```python
from build123d import *

# Parameters (mm, degrees)
SKETCH1_W                    = 3.175
SKETCH1_H                    = 244
BASE_FLANGE1_DEPTH           = 15
EDGE_FLANGE1_STRIP_W         = 14.1732
EDGE_FLANGE1_STRIP_H         = 3.175
EDGE_FLANGE1_STRIP_CUT_DEPTH = 244
EDGE_FLANGE1_DEPTH           = 244


# Sheet-metal steps are written as plain solids
with BuildPart() as part:
    # Sketch1 → Base-Flange1 (new body)
    with BuildSketch(Plane(origin=(0, 0, 0), x_dir=(0, 0, -1), z_dir=(1, 0, 0))):
        with Locations((1.5875, 0)):
            Rectangle(SKETCH1_W, SKETCH1_H)
    extrude(amount=BASE_FLANGE1_DEPTH)

    # Edge-Flange1 strip (across the edge) → Edge-Flange1 strip cut (cut)
    with BuildSketch(Plane.XZ.offset(-122)):
        with Locations((-3.175, -1.5875)):
            Rectangle(EDGE_FLANGE1_STRIP_W, EDGE_FLANGE1_STRIP_H)
    extrude(amount=EDGE_FLANGE1_STRIP_CUT_DEPTH, mode=Mode.SUBTRACT)

    # Edge-Flange1 section (across the edge) → Edge-Flange1 (add)
    with BuildSketch(Plane.XZ.offset(-122)):
        with BuildLine():
            Line((0, 0.7366), (0, 11.825))
            Line((0, 11.825), (3.175, 11.825))
            Line((3.175, 11.825), (3.175, 0.7366))
            ThreePointArc((3.175, 0.7366), (3.390745145, 0.215745145), (3.9116, 0))
            Line((3.9116, 0), (3.9116, -3.175))
            ThreePointArc((3.9116, -3.175), (1.145681115, -2.029318885), (0, 0.7366))
        make_face()
    extrude(amount=EDGE_FLANGE1_DEPTH)


solid = part.part
```
Can you work these out from the model? Positions are in its coordinate system, mm. A direction names the side the tool comes from. Coordinates: 2 decimals unless noted, no trailing zeros. Loops run counter-clockwise (first coordinate to the right, second up) from the corner with the lowest first, then second, coordinate; pieces in that order, holes last.
1) Imagine slicing it at A-A on y = -37. List the corners of the cut face in (x, z) for me (3 decimals), plus the area to 3 significant figures.
2) Which directions (+Z, -Z, +X, -X, +Y, -Y) give clear straight access to the entire face, cutting with the end or side of a thin tool? Please do faces 1 (the flat face through (3.175, 2, 6)), 2 (the flat face through (3, 122, 3)).
3) For pin 1 (1 mm diameter, centred on y = -24.5, z = 7.5, fed in from +X) (3 decimals); pin 2 (1.5 mm diameter, centred on x = 11, y = 52, fed in from +Z), each with a flat end and sliding along its axis, tell me the tip position at first contact or that it passes through.
4) I need wall thicknesses on probe 1 along X at (y, z) = (30.5, 9.5) (3 decimals); probe 2 along Z at (x, y) = (5.5, 48.5) (3 decimals); probe 3 along X at (y, z) = (54.5, -1.75). Which ranges of each line are inside material? Lowest first, please.
5) Imagine slicing it at B-B on x = 7.25. List the corners of the cut face in (y, z) for me (3 decimals), plus the area to 3 significant figures.
6) Imagine slicing it at C-C on z = 7. List the corners of the cut face in (x, y) for me (3 decimals).
Completed:
1. outline: (0, 0.737) arc R3.912 ccw to (3.912, -3.175) - (15, -3.175) - (15, 0) - (3.912, 0) arc R0.737 cw to (3.175, 0.737) - (3.175, 11.825) - (0, 11.825) - close
1. area: 82.0 mm2
2. face 1: +Z, +X, +Y, -Y
2. face 2: +Z, -Z, +X, -X, +Y
3. pin 1: stops at x = 3.175
3. pin 2: stops at z = 0
4. probe 1: x = 0 to 3.175
4. probe 2: z = -3.175 to 0
4. probe 3: x = 0.89 to 15
5. outline: (-122, -3.175) - (122, -3.175) - (122, 0) - (-122, 0) - close
5. area: 775 mm2
6. outline: (0, -122) - (3.175, -122) - (3.175, 122) - (0, 122) - close
